Job drawing, mm, ordinate dimensions from the low corner. One solid piece. Coordinates: 2 decimals unless noted, no trailing zeros. Write each loop counter-clockwise with the first axis right and the second up, starting at its lowest first coordinate (ties: lowest second). Pieces come first, ordered by that corner, then holes.
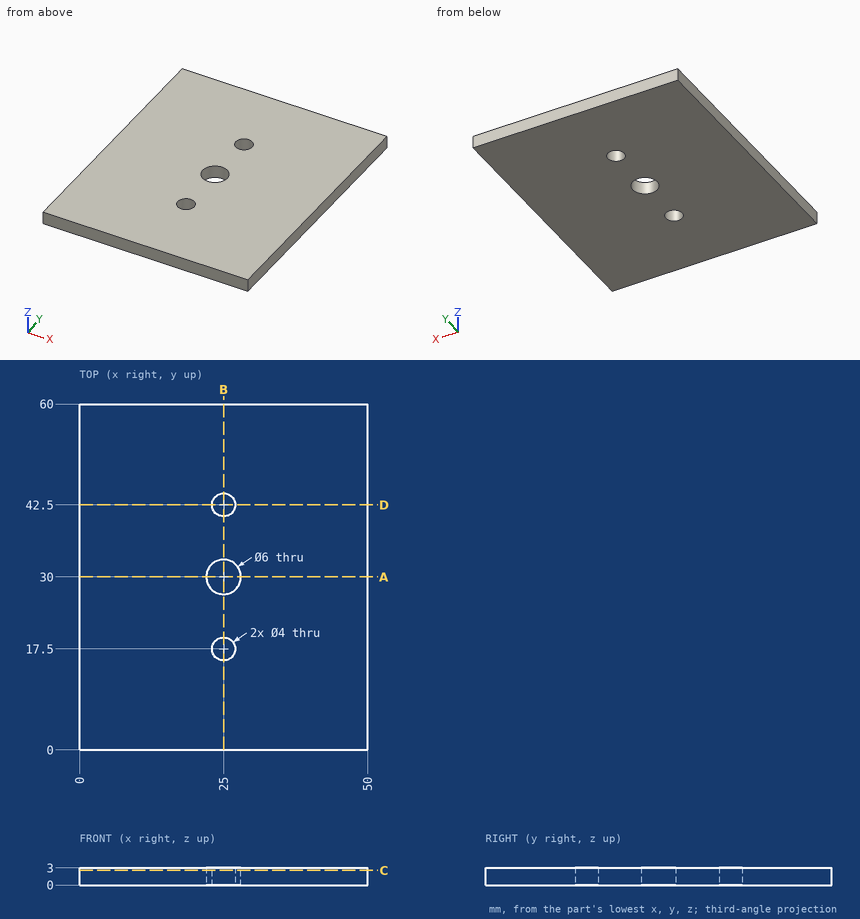
1. Flat gauge pin, fed straight in: pin 1 (3.5 mm diameter, centred on x = 25, y = 42.5, fed in from -Z). Where does the tip first touch, or does it go through?
Computed values:
pin 1: passes through
2. Probe line 1 along Y through (x, z) = (25, 1.1); line 2 along Y through (x, z) = (24.5, 0.35). List the from-to ranges inside material, lowest first.
Computed values:
line 1: y = 0 to 15.5, 19.5 to 27, 33 to 40.5, 44.5 to 60
line 2: y = 0 to 15.56, 19.44 to 27.04, 32.96 to 40.56, 44.44 to 60
3. Saw through at D-D on y = 42.5. List the corners of the cut face in (x, z), plus the area to 3 significant figures.
Computed values:
outline: (0, 0) - (23, 0) - (23, 3) - (0, 3) - close; (27, 0) - (50, 0) - (50, 3) - (27, 3) - close
area: 138 mm2
4. Saw through at C-C on z = 2.55. List the corners of the cut face in (x, y), plus the area to 3 significant figures.
Computed values:
outline: (0, 0) - (50, 0) - (50, 60) - (0, 60) - close; hole circle Ø6 at (25, 30); hole circle Ø4 at (25, 17.5); hole circle Ø4 at (25, 42.5)
area: 2,950 mm2
5. Saw through at B-B on x = 25. List the corners of the cut face in (y, z), plus the area to 3 significant figures.
Computed values:
outline: (0, 0) - (15.5, 0) - (15.5, 3) - (0, 3) - close; (19.5, 0) - (27, 0) - (27, 3) - (19.5, 3) - close; (33, 0) - (40.5, 0) - (40.5, 3) - (33, 3) - close; (44.5, 0) - (60, 0) - (60, 3) - (44.5, 3) - close
area: 138 mm2
6. Saw through at A-A on y = 30. List the corners of the cut face in (x, z).
Computed values:
outline: (0, 0) - (22, 0) - (22, 3) - (0, 3) - close; (28, 0) - (50, 0) - (50, 3) - (28, 3) - close
